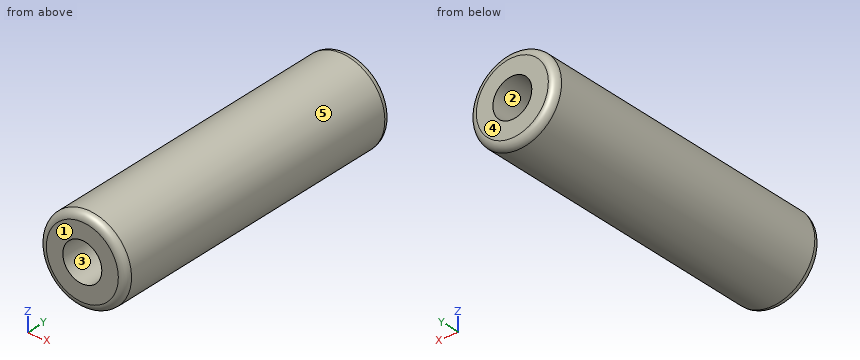
from build123d import *

# Parameters (mm, degrees)
BOSS_EXTRUDE1_DEPTH      = 10.99
BOSS_EXTRUDE1_DEPTH_BACK = 10.99
SKETCH1_R                = 3
FILLET1_R                = 0.5


with BuildPart() as part:
    # Sketch1 → Boss-Extrude1 (new, two sides: drawn at the far end of the back side and taken through both)
    with BuildSketch(Plane(origin=(0, 0, 0), x_dir=(1, 0, 0), z_dir=(0, 1, 0)).offset(-BOSS_EXTRUDE1_DEPTH_BACK)):
        with Locations(Location((0, 0, 0), (0, 0, 270))):
            Circle(SKETCH1_R)
    extrude(amount=BOSS_EXTRUDE1_DEPTH + BOSS_EXTRUDE1_DEPTH_BACK)

    # Sketch3 → 6-32 Tapped Hole1 (revolve, cut)
    with BuildSketch(Plane(origin=(0, 10.99, 0), x_dir=(0, 0, 1), z_dir=(1, 0, 0))):
        Polygon((0, 0), (0, 8.81269403), (1.35255, 8), (1.35255, 0), align=None)
    f_6_32_tapped_hole1 = revolve(axis=Axis((0, 17.34, 0), (0, -1, 0)), mode=Mode.SUBTRACT)

    # Fillet1
    fillet1_edges = [part.edges().sort_by_distance(p)[0] for p in [
        (0, -10.99, -3),
        (0, 10.99, -3),
    ]]
    fillet(fillet1_edges, radius=FILLET1_R)

    # Mirror1: 6-32 Tapped Hole1 across plane
    add(f_6_32_tapped_hole1.mirror(Plane.ZX), mode=Mode.SUBTRACT)


solid = part.part
Check sheet for the modelled part. Datum: model origin and axes. Units: mm. Face numbers are marked on the shaded views. A direction names the side the tool comes from. Round coordinates to 2 decimals unless told otherwise and drop trailing zeros. Loops run counter-clockwise (first coordinate to the right, second up) from the corner with the lowest first, then second, coordinate; pieces in that order, holes last. Notation, with made-up numbers: (68.5, -30.5) -> (103.5, -30.5) arc R13 ccw to (103.5, -14.5) -> close; hole circle Ø8 at (87.5, -8). An arc over 180 degrees is marked (long way). Put each result on its own line as item: value. Start each with the question number.
1. Section check B-B (y = 1.25). Enter the section's corners in (x, z).
2. Section check A-A (y = 4). Enter the section's corners in (x, z).
3. Access from +Z, -Z, +X, -X, +Y, -Y to the whole of each face (thin tool, end or side, straight path). Record for the marked faces 1 and 2.
4. Section check C-C (y = -2.75). Enter the section's corners in (x, z), plus the area to 3 significant figures.
5. Gauge pin test, flat ends, axial feed: pin 1 (2 mm diameter, centred on x = 2, y = -5.5, fed in from -Z); pin 2 (2.5 mm diameter, centred on x = 0, z = 0, fed in from -Y); pin 3 (1.5 mm diameter, centred on x = 1.5, y = -4.5, fed in from -Z). Record the tip position at first contact, or that the pin passes through.
6. Draft check along X on the marked faces 3, 4 and 5. Enter one of: +X half, -X half, draft (parallel to the pull), parting line (faces both ways), or undercut.
7. Scan lines: probe 1 along X at (y, z) = (9.25, 0); probe 2 along X at (y, z) = (-2.25, 0.25); probe 3 along Z at (x, y) = (-0.7, 9.5). Record each from-to range of solid material in increasing order.
Findings:
1. outline: circle Ø6 at (0, 0)
2. outline: circle Ø6 at (0, 0); hole circle Ø2.71 at (0, 0)
3. face 1: +Z, -Z, +X, -X, -Y
3. face 2: +Y
4. outline: circle Ø6 at (0, 0); hole circle Ø1.91 at (0, 0)
4. area: 25.4 mm^2
5. pin 1: stops at z = -2.83
5. pin 2: stops at y = -2.93
5. pin 3: stops at z = -2.9
6. face 3: undercut
6. face 4: draft
6. face 5: parting line
7. probe 1: x = -3 to -1.35, 1.35 to 3
7. probe 2: x = -2.99 to 2.99
7. probe 3: z = -2.92 to -1.16, 1.16 to 2.92
